from build123d import *

# Parameters (mm, degrees)
SKETCH1_W            = 160
SKETCH1_H            = 50
BOSS_EXTRUDE1_DEPTH  = 3
SKETCH2_W            = 160
SKETCH2_H            = 1
CUT_EXTRUDE1_DEPTH   = 1.5
SKETCH3_W            = 5
SKETCH3_H            = 65
BOSS_EXTRUDE2_DEPTH  = 1.5
SKETCH4_W            = 160
SKETCH4_H            = 3
BOSS_EXTRUDE3_DEPTH  = 5
SKETCH5_W            = 3
SKETCH5_H            = 47
BOSS_EXTRUDE4_DEPTH  = 5
SKETCH6_W            = 160
SKETCH6_H            = 5
BOSS_EXTRUDE5_DEPTH  = 2
SKETCH7_W            = 2
SKETCH7_H            = 65
BOSS_EXTRUDE6_DEPTH  = 2
FILLET1_R            = 2
SKETCH8_W            = 5
SKETCH8_H            = 160
BOSS_EXTRUDE7_DEPTH  = 2
SKETCH9_W            = 10
SKETCH9_H            = 47
BOSS_EXTRUDE8_DEPTH  = 5
BOSS_EXTRUDE9_DEPTH  = 2.5
BOSS_EXTRUDE10_DEPTH = 1.5
SKETCH12_W           = 4.967149052
SKETCH12_H           = 65
BOSS_EXTRUDE11_DEPTH = 0.5


with BuildPart() as part:
    # Sketch1 → Boss-Extrude1 (new body)
    with BuildSketch(Plane(origin=(0, 0, 0), x_dir=(0, 0, -1), z_dir=(1, 0, 0))):
        Rectangle(SKETCH1_W, SKETCH1_H)
    extrude(amount=BOSS_EXTRUDE1_DEPTH)

    # Sketch2 → Cut-Extrude1 (cut)
    with BuildSketch(Plane(origin=(3, 0, 0), x_dir=(0, 0, -1), z_dir=(1, 0, 0))):
        with Locations((0, -17.5)):
            Rectangle(SKETCH2_W, SKETCH2_H)
        with Locations((0, -6.5)):
            Rectangle(SKETCH2_W, SKETCH2_H)
        with Locations((0, 4.5)):
            Rectangle(SKETCH2_W, SKETCH2_H)
        with Locations((0, 15.5)):
            Rectangle(SKETCH2_W, SKETCH2_H)
    extrude(amount=-CUT_EXTRUDE1_DEPTH, mode=Mode.SUBTRACT)

    # Sketch3 → Boss-Extrude2 (add, symmetric)
    with BuildSketch(Plane(origin=(3, 0, 0), x_dir=(0, 0, -1), z_dir=(1, 0, 0))):
        with Locations((-77.5, 7.5)):
            Rectangle(SKETCH3_W, SKETCH3_H)
        with Locations((-42.5, 7.5)):
            Rectangle(SKETCH3_W, SKETCH3_H)
        with Locations((12.5, 7.5)):
            Rectangle(SKETCH3_W, SKETCH3_H)
        with Locations((67.5, 7.5)):
            Rectangle(SKETCH3_W, SKETCH3_H)
    extrude(amount=BOSS_EXTRUDE2_DEPTH, both=True)

    # Sketch4 → Boss-Extrude3 (add)
    with BuildSketch(Plane.ZY):
        with Locations((0, -23.5)):
            Rectangle(SKETCH4_W, SKETCH4_H)
    extrude(amount=BOSS_EXTRUDE3_DEPTH)

    # Sketch5 → Boss-Extrude4 (add)
    with BuildSketch(Plane.ZY):
        with Locations((78.5, 1.5)):
            Rectangle(SKETCH5_W, SKETCH5_H)
    extrude(amount=BOSS_EXTRUDE4_DEPTH)

    # Sketch6 → Boss-Extrude5 (add)
    with BuildSketch(Plane.ZY):
        with Locations((0, 29.5)):
            Rectangle(SKETCH6_W, SKETCH6_H)
        with Locations((0, 37.5)):
            Rectangle(SKETCH6_W, SKETCH6_H)
    extrude(amount=-BOSS_EXTRUDE5_DEPTH)

    # Sketch7 → Boss-Extrude6 (add)
    with BuildSketch(Plane(origin=(4.5, 0, 0), x_dir=(0, 0, -1), z_dir=(1, 0, 0))):
        with Locations((-44, 7.5)):
            Rectangle(SKETCH7_W, SKETCH7_H)
        with Locations((11, 7.5)):
            Rectangle(SKETCH7_W, SKETCH7_H)
        with Locations((66, 7.5)):
            Rectangle(SKETCH7_W, SKETCH7_H)
    extrude(amount=BOSS_EXTRUDE6_DEPTH)

    # Fillet1
    fillet1_edges = [part.edges().sort_by_distance(p)[0] for p in [
        (6.5, 40, -66),
        (6.5, 40, -11),
        (6.5, 40, 44),
    ]]
    fillet(fillet1_edges, radius=FILLET1_R)

    # Sketch8 → Boss-Extrude7 (add)
    with BuildSketch(Plane(origin=(0, 40, 0), x_dir=(1, 0, 0), z_dir=(0, 1, 0))):
        with Locations((2.5, 0)):
            Rectangle(SKETCH8_W, SKETCH8_H)
    extrude(amount=BOSS_EXTRUDE7_DEPTH)

    # Sketch9 → Boss-Extrude8 (add)
    with BuildSketch(Plane.ZY):
        with Locations((-80, 1.5)):
            Rectangle(SKETCH9_W, SKETCH9_H)
    extrude(amount=BOSS_EXTRUDE8_DEPTH)

    # Sketch10 → Boss-Extrude9 (add)
    with BuildSketch(Plane(origin=(2, 0, 0), x_dir=(0, 0, -1), z_dir=(1, 0, 0))):
        Polygon((-75, 40), (-75, 35), (-67, 40), align=None)
    extrude(amount=BOSS_EXTRUDE9_DEPTH)

    # Sketch11 → Boss-Extrude10 (add)
    with BuildSketch(Plane(origin=(3, 0, 0), x_dir=(0, 0, -1), z_dir=(1, 0, 0))):
        Polygon((-45, 25), (-75, 25), (-75, 20), (-71, 22), (-49, 22), (-45, 20), align=None)
    extrude(amount=BOSS_EXTRUDE10_DEPTH)

    # Sketch12 → Boss-Extrude11 (add)
    with BuildSketch(Plane(origin=(4.5, 0, 0), x_dir=(0, 0, -1), z_dir=(1, 0, 0))):
        with Locations((-77.516425474, 7.5)):
            Rectangle(SKETCH12_W, SKETCH12_H)
    extrude(amount=BOSS_EXTRUDE11_DEPTH)


solid = part.part
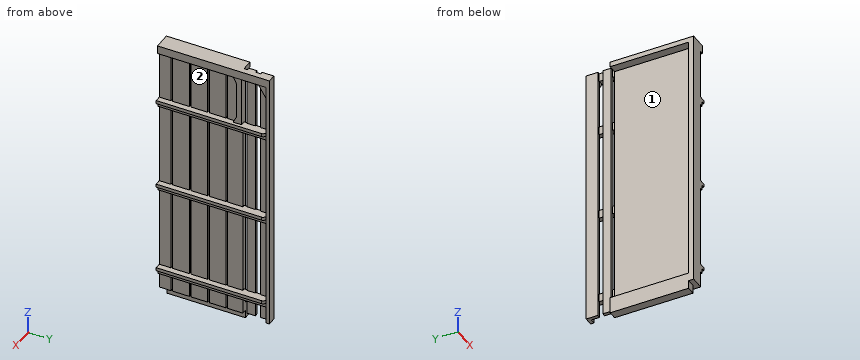
Here's how the part is built. I have some questions about the finished solid (model axes, mm). Face numbers are marked on the shaded views. A direction names the side the tool comes from. Round coordinates to 2 decimals unless told otherwise and drop trailing zeros. Write each loop counter-clockwise with the first axis right and the second up, starting at its lowest first coordinate (ties: lowest second). Pieces come first, ordered by that corner, then holes.
1. Suppose I cut it at A-A (z = -3.5). State how many separate pieces and enclosed holes the cut face has, and give its area (3 significant figures).
2. I need wall thicknesses on L1, parallel to Z at x = 4.75, y = 4; L2, parallel to Z at x = 6, y = -9; L3, parallel to Z at x = -2.25, y = -12. Which ranges of each line are inside material? Lowest first, please.
3. Suppose I cut it at B-B (x = -2.75). List the corners of the cut face in (y, z) for me.
4. For the marked faces 1 and 2, which set-ups out of +Z, -Z, +X, -X, +Y, -Y let a thin tool reach every point of the face, with its end or its side?
5. Will these pins go through, and if not, where does the flat tip stop? pin 1 Ø2.5 at (y, z) = (-7.5, -68.5) entering from +X; pin 2 Ø0.6 at (y, z) = (26.5, 76.5) entering from -X; pin 3 Ø10 at (y, z) = (9, -68) entering from +X; pin 4 Ø8 at (y, z) = (-15.5, -43) entering from -X.
Answer sheet:
1. separate pieces: 3
1. enclosed holes: 0
1. area: 189 mm2
2. L1: z = -67 to -65, -12 to -10, 43 to 45, 75.03 to 80
2. L2: z = -67 to -65, -12 to -10, 43 to 45
2. L3: z = -85 to -75, 77 to 80
3. outline: (-25, -80) - (-22, -80) - (-22, -85) - (25, -85) - (25, -75) - (-22, -75) - (-22, 77) - (25, 77) - (25, 80) - (-25, 80) - close
4. face 1: -X, +Y
4. face 2: +X, -Y
5. pin 1: stops at x = 4.5
5. pin 2: stops at x = 1.5
5. pin 3: stops at x = 6.5
5. pin 4: stops at x = 0
